from build123d import *

# Parameters (mm, degrees)
F1_DEPTH    = 15
F2_T1_DEPTH = 32.7362862295
F3_R        = 7


# Not quite as in the source:
# - a fillet or chamfer that OpenCascade refuses, or shapes differently, is made with other operations: its cross-section is extruded or revolved along the edge and cut away or added


with BuildPart() as f1:
    # F0 (on Front) → F1 (new body)
    with BuildSketch(Plane.XZ):
        Polygon((-14, 0), (14, 0), (14, 2), (0, 5), (-14, 2), align=None)
    extrude(amount=F1_DEPTH)

    # F2: fillet of radius 5 on 2 edges, made by hand

    # F2_s2 → F2_t1 (cut)
    with BuildSketch(Plane.XZ.offset(-8.8681431148)):
        with BuildLine():
            ThreePointArc((-10.5314833016, 2.7432535782), (-12.5855065639, 1.7759313526), (-14, 0))
            Line((-14, 0), (-14, 2))
            Line((-14, 2), (-10.5314833016, 2.7432535782))
        make_face()
        with BuildLine():
            ThreePointArc((14, 0), (12.5855065639, 1.7759313526), (10.5314833016, 2.7432535782))
            Line((10.5314833016, 2.7432535782), (14, 2))
            Line((14, 2), (14, 0))
        make_face()
    extrude(amount=F2_T1_DEPTH, mode=Mode.SUBTRACT)

    # F3
    f3_edges = [f1.edges().sort_by_distance(p)[0] for p in [
        (0, -7.5, 5),
    ]]
    fillet(f3_edges, radius=F3_R)


solid = f1.part
The listing builds one solid part. Answer for the finished solid, in the listing's coordinates (mm). Round coordinates to 2 decimals unless told otherwise and drop trailing zeros. Loops run counter-clockwise (first coordinate to the right, second up) from the corner with the lowest first, then second, coordinate; pieces in that order, holes last. Notation, with made-up numbers: M -0.75,67 L 22.25,67 A28 ccw 22.25,92 Z; hole C -32.5,42.25 d3. An arc over 180 degrees is marked long. Write each question's results on one line, items separated by ' | '. Start each with the question number.
1) This flat-tipped pin is pushed along its axis until it touches: pin 1 (6 mm diameter, centred on x = -10.5, y = -5, fed in from +Z). Where does it stop, or does it pass through?
2) Find section C-C on x = 11.5. Write down the section's boundary in (y, z), plus the area to 3 significant figures.
3) Find section A-A on y = -10.5. Write down the section's boundary in (x, z), plus the area to 3 significant figures.
4) Find section B-B on z = 0.4. Write down the section's boundary in (x, y), plus the area to 3 significant figures.
5) Straight lines are drawn through the part: probe 1 along Z at (x, y) = (10.5, -12.75); probe 2 along X at (y, z) = (-3.25, 1.9); probe 3 along X at (y, z) = (-10, 2.05). For each, find the intervals that lie inside material, in ascending order.
6) Determine the mould class of faces 1 (the flat face through (0, -7, 0)), 2 (the flat face through (0, -15, 2)), 3 (the cylindrical face through (12.611, -7.395, 1.756)) for opening direction Z: pulls with the +Z half, pulls with the -Z half, needs draft (parallel to the pull), parting line crosses it, or undercut.
Final values:
1) pin 1: z = 3.39
2) outline: M -15,0 L 0,0 L 0,2.43 L -15,2.43 Z | area: 36.4 mm²
3) outline: M -14,0 L 14,0 A5 ccw 10.53,2.74 L 1.47,4.69 A7 ccw -1.47,4.69 L -10.53,2.74 A5 ccw Z | area: 94.0 mm²
4) outline: M -13.79,-15 L 13.79,-15 L 13.79,0 L -13.79,0 Z | area: 414 mm²
5) probe 1: 0 to 2.75 | probe 2: -12.42 to 12.42 | probe 3: -12.2 to 12.2
6) face 1: pulls with the -Z half | face 2: needs draft | face 3: pulls with the +Z half
